The drawing under review shows one solid part. Ordinate dimensions are in mm from its lowest x, y, z. A direction names the side the tool comes from. Give positions to 0.01 mm unless a question says otherwise; leave off trailing zeros. Loops run counter-clockwise (first coordinate to the right, second up) from the corner with the lowest first, then second, coordinate; pieces in that order, holes last. Notation, with made-up numbers: (44, 43.25) - (80, 43.25) arc R17 ccw to (80, 54.25) - close; hole circle Ø6 at (35, -24.5). An arc over 180 degrees is marked (long way). Write each question's results on one line, items separated by ' | '.
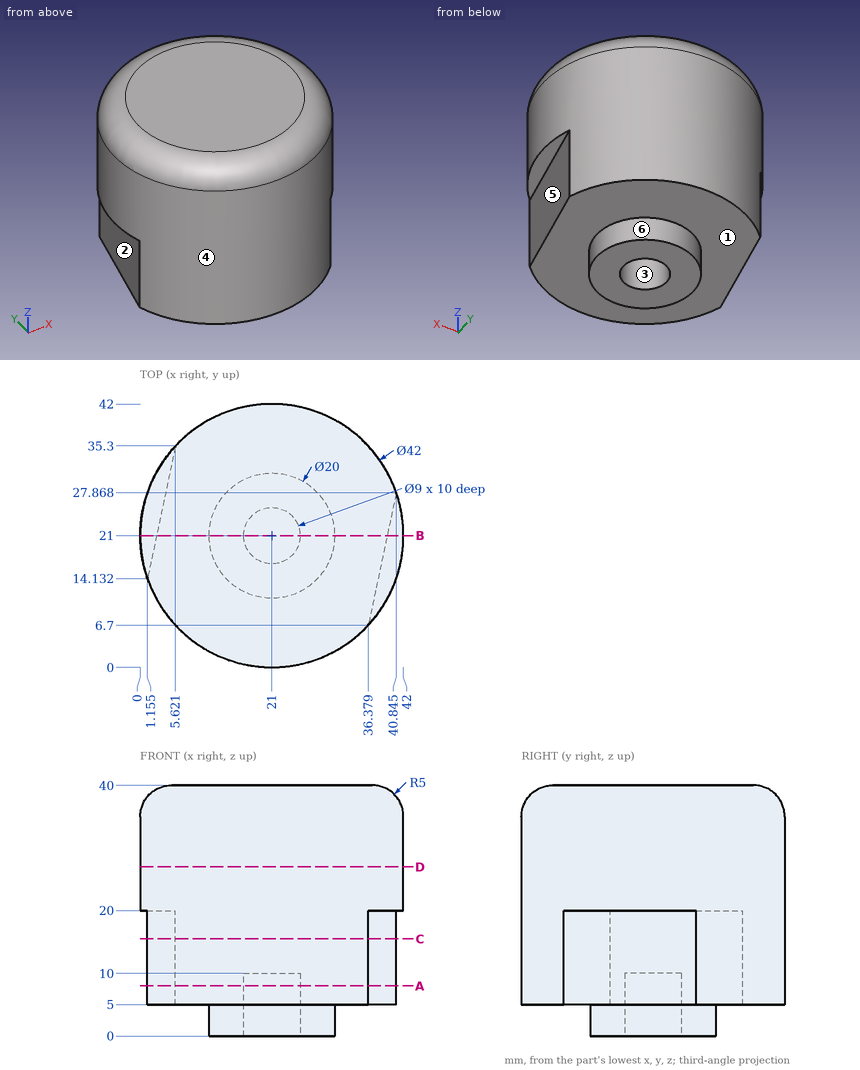
(1) Insertion check: P1, Ø1, axis at y = 6, z = 30, coming from the +X side; P2, Ø4, axis at y = 36, z = 21.5, coming from the -X side; P3, Ø2, axis at x = 20.5, z = 8.5, coming from the -Y side. Each pin has a flat end and moves straight along its axis. Give the tip position at first contact, or say it passes through.
Answers below:
P1: x = 36.19 | P2: x = 4.51 | P3: y = 0
(2) Wall thickness on line 1 along Y through (x, z) = (21, 4); line 2 along Z through (x, y) = (32, 19); line 3 along Y through (x, z) = (20.5, 20): over which ranges is each line inside the solid? List them lowest first. Write a range as from..to.
Answers below:
line 1: 11..16.5, 25.5..31 | line 2: 5..40 | line 3: 0.01..41.99
(3) Take a section at D-D on z = 27. Give the boundary of the cut face in (x, y).
Answers below:
outline: circle Ø42 at (21, 21)
(4) Draft analysis for pull direction X (two halves, no side actions). For the marked faces 1, 2 and 3, state which applies: pulls with the +X half, pulls with the -X half, needs draft (parallel to the pull), parting line crosses it, or undercut.
Answers below:
face 1: needs draft | face 2: pulls with the -X half | face 3: undercut
(5) Take a section at C-C on z = 15.5. Give the boundary of the cut face in (x, y) (1 decimal), plus the area to 3 significant figures.
Answers below:
outline: (1.2, 14.1) arc R21 ccw to (36.4, 6.7) - (40.8, 27.9) arc R21 ccw to (5.6, 35.3) - close | area: 1,300 mm2
(6) Take a section at B-B on y = 21. Give the boundary of the cut face in (x, z).
Answers below:
outline: (0, 20) - (2.6, 20) - (2.6, 5) - (11, 5) - (11, 0) - (16.5, 0) - (16.5, 10) - (25.5, 10) - (25.5, 0) - (31, 0) - (31, 5) - (39.4, 5) - (39.4, 20) - (42, 20) - (42, 35) arc R5 ccw to (37, 40) - (5, 40) arc R5 ccw to (0, 35) - close
(7) Take a section at A-A on z = 8. Give the boundary of the cut face in (x, y) (1 decimal).
Answers below:
outline: (1.2, 14.1) arc R21 ccw to (36.4, 6.7) - (40.8, 27.9) arc R21 ccw to (5.6, 35.3) - close; hole circle Ø9 at (21, 21)
(8) Tool access review of the marked faces 4, 5 and 6: name each direction out of +Z, -Z, +X, -X, +Y, -Y from which nothing blocks a thin tool from reaching the whole face with its end or side.
Answers below:
face 4: +Z, -Z | face 5: -Z, +X, -Y | face 6: -Z
